Source: CAD feature listing. Evaluate the final solid. Frame: model axes, mm. Face numbers are marked on the shaded views. A direction names the side the tool comes from. Coordinates: 2 decimals unless noted, no trailing zeros. Write each loop counter-clockwise with the first axis right and the second up, starting at its lowest first coordinate (ties: lowest second). Pieces come first, ordered by that corner, then holes. Notation, with made-up numbers: M -21.5,-10.5 L 13.5,-10.5 A22 ccw 13.5,-4.5 Z; hole C 88.25,23.5 d6. An arc over 180 degrees is marked long. Write item = value, one per line. Start each with the question number.
1. Section query C-C (y = 22.6). Output: boundary loops of the cut face in (x, z).
2. Section query B-B (z = 30). Output: boundary loops of the cut face in (x, y), then the cut area to 3 significant figures.
3. Pull-direction query (Z, two-part tool) for the marked faces 1, 2 and 3; classes: pulls with the +Z half, pulls with the -Z half, needs draft (parallel to the pull), parting line crosses it, or undercut.
4. Line query: line 1 along Y through (x, z) = (-34.5, 62); line 2 along Z through (x, y) = (-34, -7); line 3 along X through (y, z) = (24.5, 51.5). Output: solid intervals per line, ascending.
5. Access query for the marked faces 4, 5, 6 and 7. Directions: +Z, -Z, +X, -X, +Y, -Y. A direction counts if a zero-diameter tool reaches every point of the face in a straight line with its end or side. Return the directions, or none.
6. Section query A-A (y = -32). Output: boundary loops of the cut face in (x, z).
7. Section query D-D (z = 98.5). Output: boundary loops of the cut face in (x, y), then the cut area to 3 significant figures.
8. Pin query (flat end, axial travel): pin 1 Ø8 at (y, z) = (-22.6, 39.4) entering from -X; pin 2 Ø10 at (x, y) = (-36.5, 7) entering from +Z; pin 3 Ø4 at (x, y) = (-46, -10.5) entering from -Z; pin 4 Ø23 at (y, z) = (0, 62) entering from +X. Return the tip coordinate at first contact, or that it passes through.
```python
from build123d import *

# Parameters (mm, degrees)
F_01_FLANGE_DEPTH    = 12
SKETCH_2_R           = 16
F_02_BOSS_UP_DEPTH   = 10
SKETCH_3_R           = 16
F_03_BOSS_LO_DEPTH   = 22
SKETCH_4_R           = 9
F_04_BORE_UP_DEPTH   = 10
SKETCH_5_R           = 9
F_05_BORE_LO_DEPTH   = 10
SKETCH_6_R           = 10
F_06_RV_CAVITY_DEPTH = 26
SKETCH_8_R           = 4
F_08_BOLT_0_DEPTH    = 14
SKETCH_9_R           = 4
F_08_BOLT_1_DEPTH    = 14
SKETCH_10_R          = 4
F_08_BOLT_2_DEPTH    = 14
SKETCH_11_R          = 4
F_08_BOLT_3_DEPTH    = 14
SKETCH_12_R          = 4
F_08_BOLT_4_DEPTH    = 14
SKETCH_13_R          = 4
F_08_BOLT_5_DEPTH    = 14
SKETCH_14_R          = 2.5
F_09_DOWEL_0_DEPTH   = 14
SKETCH_15_R          = 2.5
F_09_DOWEL_1_DEPTH   = 14


with BuildPart() as part:
    # 草图1 → 01_FLANGE (new body)
    with BuildSketch(Plane(origin=(-42, 0, 0), x_dir=(0, 0, -1), z_dir=(1, 0, 0))):
        with BuildLine():
            Line((-104, -40), (-62, -40))
            ThreePointArc((-62, -40), (-22, 0), (-62, 40))
            Line((-62, 40), (-104, 40))
            ThreePointArc((-104, 40), (-144, 0), (-104, -40))
        make_face()
    extrude(amount=F_01_FLANGE_DEPTH)

    # 草图2 → 02_BOSS_UP (add)
    with BuildSketch(Plane(origin=(-52, 0, 0), x_dir=(0, 0, -1), z_dir=(1, 0, 0))):
        with Locations((-104, 0)):
            Circle(SKETCH_2_R)
    extrude(amount=F_02_BOSS_UP_DEPTH)

    # 草图3 → 03_BOSS_LO (add)
    with BuildSketch(Plane(origin=(-64, 0, 0), x_dir=(0, 0, -1), z_dir=(1, 0, 0))):
        with Locations((-62, 0)):
            Circle(SKETCH_3_R)
    extrude(amount=F_03_BOSS_LO_DEPTH)

    # 草图4 → 04_BORE_UP (cut)
    with BuildSketch(Plane(origin=(-30, 0, 0), x_dir=(0, 0, -1), z_dir=(1, 0, 0))):
        with Locations((-104, 0)):
            Circle(SKETCH_4_R)
    extrude(amount=-F_04_BORE_UP_DEPTH, mode=Mode.SUBTRACT)

    # 草图5 → 05_BORE_LO (cut)
    with BuildSketch(Plane(origin=(-30, 0, 0), x_dir=(0, 0, -1), z_dir=(1, 0, 0))):
        with Locations((-62, 0)):
            Circle(SKETCH_5_R)
    extrude(amount=-F_05_BORE_LO_DEPTH, mode=Mode.SUBTRACT)

    # 草图6 → 06_RV_CAVITY (cut)
    with BuildSketch(Plane(origin=(-64, 0, 0), x_dir=(0, 0, -1), z_dir=(1, 0, 0))):
        with Locations(Location((-62, 0, 0), (0, 0, 180))):
            Circle(SKETCH_6_R)
    extrude(amount=F_06_RV_CAVITY_DEPTH, mode=Mode.SUBTRACT)

    # 草图8 → 08_BOLT_0 (cut)
    with BuildSketch(Plane(origin=(-43, 0, 0), x_dir=(0, 0, -1), z_dir=(1, 0, 0))):
        with Locations((-104, 32)):
            Circle(SKETCH_8_R)
    extrude(amount=F_08_BOLT_0_DEPTH, mode=Mode.SUBTRACT)

    # 草图9 → 08_BOLT_1 (cut)
    with BuildSketch(Plane(origin=(-43, 0, 0), x_dir=(0, 0, -1), z_dir=(1, 0, 0))):
        with Locations((-104, -32)):
            Circle(SKETCH_9_R)
    extrude(amount=F_08_BOLT_1_DEPTH, mode=Mode.SUBTRACT)

    # 草图10 → 08_BOLT_2 (cut)
    with BuildSketch(Plane(origin=(-43, 0, 0), x_dir=(0, 0, -1), z_dir=(1, 0, 0))):
        with Locations((-62, 32)):
            Circle(SKETCH_10_R)
    extrude(amount=F_08_BOLT_2_DEPTH, mode=Mode.SUBTRACT)

    # 草图11 → 08_BOLT_3 (cut)
    with BuildSketch(Plane(origin=(-43, 0, 0), x_dir=(0, 0, -1), z_dir=(1, 0, 0))):
        with Locations((-62, -32)):
            Circle(SKETCH_11_R)
    extrude(amount=F_08_BOLT_3_DEPTH, mode=Mode.SUBTRACT)

    # 草图12 → 08_BOLT_4 (cut)
    with BuildSketch(Plane(origin=(-43, 0, 0), x_dir=(0, 0, -1), z_dir=(1, 0, 0))):
        with Locations((-136, 0)):
            Circle(SKETCH_12_R)
    extrude(amount=F_08_BOLT_4_DEPTH, mode=Mode.SUBTRACT)

    # 草图13 → 08_BOLT_5 (cut)
    with BuildSketch(Plane(origin=(-43, 0, 0), x_dir=(0, 0, -1), z_dir=(1, 0, 0))):
        with Locations((-30, 0)):
            Circle(SKETCH_13_R)
    extrude(amount=F_08_BOLT_5_DEPTH, mode=Mode.SUBTRACT)

    # 草图14 → 09_DOWEL_0 (cut)
    with BuildSketch(Plane(origin=(-43, 0, 0), x_dir=(0, 0, -1), z_dir=(1, 0, 0))):
        with Locations((-126.6, 22.6)):
            Circle(SKETCH_14_R)
    extrude(amount=F_09_DOWEL_0_DEPTH, mode=Mode.SUBTRACT)

    # 草图15 → 09_DOWEL_1 (cut)
    with BuildSketch(Plane(origin=(-43, 0, 0), x_dir=(0, 0, -1), z_dir=(1, 0, 0))):
        with Locations((-39.4, -22.6)):
            Circle(SKETCH_15_R)
    extrude(amount=F_09_DOWEL_1_DEPTH, mode=Mode.SUBTRACT)


solid = part.part
```
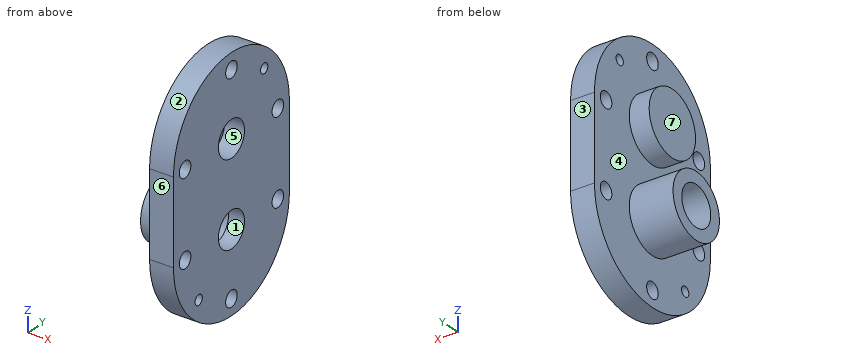
Results are:
q1.outline = M -42,29 L -30,29 L -30,124.1 L -42,124.1 Z; M -42,129.1 L -30,129.1 L -30,137 L -42,137 Z
q2.outline = M -42,-24 L -30,-24 L -30,-4 L -42,-4 Z; M -42,4 L -30,4 L -30,24 L -42,24 Z
q2.area = 480 mm^2
q3.face_1 = undercut
q3.face_2 = pulls with the +Z half
q3.face_3 = needs draft
q4.line_1 = -40 to -36, -28 to -9, 9 to 28, 36 to 40
q4.line_2 = 22.62 to 56.34, 67.66 to 98.34, 109.66 to 143.38
q4.line_3 = -42 to -30
q5.face_4 = -X
q5.face_5 = +X
q5.face_6 = +Z, -Z, +X, -X, -Y
q5.face_7 = +Z, -X, +Y, -Y
q6.outline = M -42,38 L -30,38 L -30,58 L -42,58 Z; M -42,66 L -30,66 L -30,100 L -42,100 Z; M -42,108 L -30,108 L -30,128 L -42,128 Z
q7.outline = M -52,-15.02 L -42,-15.02 L -42,-40 L -30,-40 L -30,-7.12 L -40,-7.12 L -40,7.12 L -30,7.12 L -30,40 L -42,40 L -42,15.02 L -52,15.02 Z
q7.area = 1,120 mm^2
q8.pin_1 = -42
q8.pin_2 = 143.95
q8.pin_3 = 48.44
q8.pin_4 = -30
